The model under review builds one solid part; all positions refer to its coordinate system, in mm. Face numbers are marked on the shaded views. A direction names the side the tool comes from. Give positions to 0.01 mm unless a question says otherwise; leave off trailing zeros. Order: outer loops, then holes, each group sorted by start corner. A loop starts at its lowest first (then second) coordinate and runs counter-clockwise, first axis right, second up. Notation, with made-up numbers: (19.25, 70.5) - (67.25, 70.5) arc R11 cw to (67.25, 84.5) - close; hole circle Ø2 at (-34.75, 47.5). An arc over 180 degrees is marked (long way). Answer as CSV lines item,"result". Start each with the question number.
from build123d import *

# Parameters (mm, degrees)
SKETCH1_W                 = 43
SKETCH1_H                 = 60
BOSS_EXTRUDE1_DEPTH       = 55
SKETCH2_W                 = 41.9
SKETCH2_H                 = 20.5
SKETCH2_H_2               = 20
CUT_EXTRUDE1_DEPTH        = 38
SKETCH3_W                 = 9.05
SKETCH3_H                 = 8.5
CUT_EXTRUDE2_DEPTH        = 38
BOSS_EXTRUDE5_START       = -0.874015748
BOSS_EXTRUDE5_OUTLINE_W   = 2.5
BOSS_EXTRUDE5_OUTLINE_H   = 41.9
BOSS_EXTRUDE5_OUTLINE_W_2 = 5
BOSS_EXTRUDE5_OUTLINE_H_2 = 20
BOSS_EXTRUDE5_DEPTH       = 30
SKETCH18_R                = 2.5
CUT_EXTRUDE9_DEPTH        = 10
SKETCH19_R                = 2.5
CUT_EXTRUDE10_DEPTH       = 10
SKETCH20_W                = 41.9
SKETCH20_H                = 5
CUT_EXTRUDE11_DEPTH       = 25
SKETCH21_W                = 60
SKETCH21_H                = 55
CUT_EXTRUDE12_DEPTH       = 13
SKETCH22_W                = 41.9
SKETCH22_H                = 2
BOSS_EXTRUDE6_DEPTH       = 25
FILLET4_R                 = 1
FILLET5_R                 = 1


# Read off the part's stored shape, not the designer's step: Boss-Extrude5
with BuildPart() as part:
    # Sketch1 → Boss-Extrude1 (new body)
    with BuildSketch(Plane(origin=(0, 0, 0), x_dir=(1, 0, 0), z_dir=(0, 1, 0))):
        with Locations((20.625984252, 7.362204724)):
            Rectangle(SKETCH1_W, SKETCH1_H)
    extrude(amount=BOSS_EXTRUDE1_DEPTH)

    # Sketch2 → Cut-Extrude1 (cut)
    with BuildSketch(Plane(origin=(42.125984252, 0, 0), x_dir=(0, 0, -1), z_dir=(1, 0, 0))):
        with Locations((7.362204724, 40.25)):
            Rectangle(SKETCH2_W, SKETCH2_H)
        with Locations((7.362204724, 14.5)):
            Rectangle(SKETCH2_W, SKETCH2_H_2)
    extrude(amount=-CUT_EXTRUDE1_DEPTH, mode=Mode.SUBTRACT)

    # Sketch3 → Cut-Extrude2 (cut)
    with BuildSketch(Plane(origin=(42.125984252, 0, 0), x_dir=(0, 0, -1), z_dir=(1, 0, 0))):
        with Locations((-18.112795276, 14.75)):
            Rectangle(SKETCH3_W, SKETCH3_H)
        with Locations((32.837204724, 40.25)):
            Rectangle(SKETCH3_W, SKETCH3_H)
    extrude(amount=-CUT_EXTRUDE2_DEPTH, mode=Mode.SUBTRACT)

    # Boss-Extrude5 outline → Boss-Extrude5 (add)
    with BuildSketch(Plane.YZ.offset(BOSS_EXTRUDE5_START)):
        with Locations((5.75, -7.362204724)):
            Rectangle(BOSS_EXTRUDE5_OUTLINE_W, BOSS_EXTRUDE5_OUTLINE_H)
        with Locations((4.5, -47.362204724)):
            Rectangle(BOSS_EXTRUDE5_OUTLINE_W_2, BOSS_EXTRUDE5_OUTLINE_H_2)
        with Locations((4.5, 32.637795276)):
            Rectangle(BOSS_EXTRUDE5_OUTLINE_W_2, BOSS_EXTRUDE5_OUTLINE_H_2)
    extrude(amount=BOSS_EXTRUDE5_DEPTH)

    # Sketch18 → Cut-Extrude9 (cut)
    with BuildSketch(Plane(origin=(29.125984252, 0, 0), x_dir=(0, 0, -1), z_dir=(1, 0, 0))):
        with Locations((-17.437795276, 45.5)):
            Circle(SKETCH18_R)
        with Locations((-17.437795276, 35.5)):
            Circle(SKETCH18_R)
    extrude(amount=-CUT_EXTRUDE9_DEPTH, mode=Mode.SUBTRACT)

    # Sketch19 → Cut-Extrude10 (cut)
    with BuildSketch(Plane(origin=(29.125984252, 0, 0), x_dir=(0, 0, -1), z_dir=(1, 0, 0))):
        with Locations((32.162204724, 19.5)):
            Circle(SKETCH19_R)
        with Locations((32.162204724, 9.5)):
            Circle(SKETCH19_R)
    extrude(amount=-CUT_EXTRUDE10_DEPTH, mode=Mode.SUBTRACT)

    # Sketch20 → Cut-Extrude11 (cut)
    with BuildSketch(Plane(origin=(29.125984252, 0, 0), x_dir=(0, 0, -1), z_dir=(1, 0, 0))):
        with Locations((7.362204724, 4.5)):
            Rectangle(SKETCH20_W, SKETCH20_H)
    extrude(amount=-CUT_EXTRUDE11_DEPTH, mode=Mode.SUBTRACT)

    # Sketch21 → Cut-Extrude12 (cut)
    with BuildSketch(Plane(origin=(42.125984252, 0, 0), x_dir=(0, 0, -1), z_dir=(1, 0, 0))):
        with Locations((7.362204724, 27.5)):
            Rectangle(SKETCH21_W, SKETCH21_H)
    extrude(amount=-CUT_EXTRUDE12_DEPTH, mode=Mode.SUBTRACT)

    # Sketch22 → Boss-Extrude6 (add)
    with BuildSketch(Plane(origin=(4.125984252, 0, 0), x_dir=(0, 0, -1), z_dir=(1, 0, 0))):
        with Locations((7.362204724, 3)):
            Rectangle(SKETCH22_W, SKETCH22_H)
    extrude(amount=BOSS_EXTRUDE6_DEPTH)

    # Fillet4
    fillet4_edges = [part.edges().sort_by_distance(p)[0] for p in [
        (29.125984252, 44.5, -32.837204724),
        (29.125984252, 36, -32.837204724),
        (16.625984252, 36, -28.312204724),
        (16.625984252, 44.5, -28.312204724),
        (16.625984252, 44.5, -37.362204724),
        (16.625984252, 36, -37.362204724),
    ]]
    fillet(fillet4_edges, radius=FILLET4_R)

    # Fillet5
    fillet5_edges = [part.edges().sort_by_distance(p)[0] for p in [
        (29.125984252, 10.5, 18.112795276),
        (16.625984252, 10.5, 22.637795276),
        (16.625984252, 10.5, 13.587795276),
    ]]
    fillet(fillet5_edges, radius=FILLET5_R)


solid = part.part
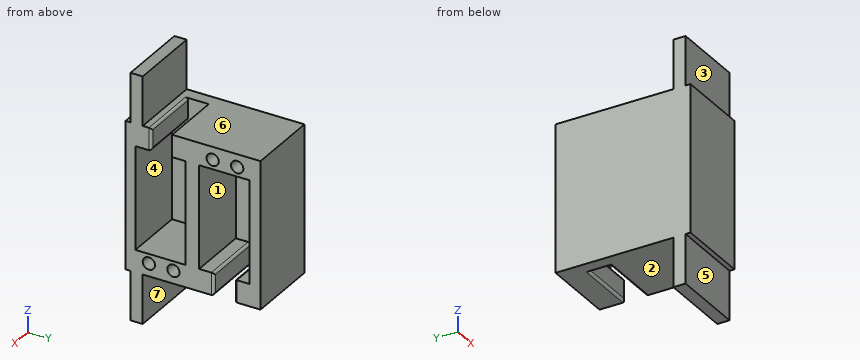
Item 1: Take a section at A-A on y = 5. Write out the cut boundary in (x, z).
Item 2: For line 1 along Y through (x, z) = (12, -20); line 2 along Z through (x, y) = (13, 21.5); line 3 along Z through (x, y) = (25, 9), list the stretches that pass through material, from the lowest coordinate up.
Item 3: Mouldability with a two-part tool opening along Y and no side actions: class the marked faces 1, 2 and 3 as released by +Y, released by -Y, zero draft, split by the parting line, or undercut.
Item 4: Clearance check with flat-ended pins moving along their axes: pin 1 (5 mm diameter, centred on x = 9.5, z = 2.5, fed in from -Y); pin 2 (6 mm diameter, centred on y = 7.5, z = 5.5, fed in from +X); pin 3 (10 mm diameter, centred on x = 10.5, y = 38.5, fed in from -Z); pin 4 (6 mm diameter, centred on x = 13, z = 35.5, fed in from +Y). State where each tip first meets the part, or that it passes through.
Item 5: Take a section at D-D on x = 27. Count the separate pieces of the cut face and the enclosed holes in it, and give its area (3 significant figures).
Item 6: Machinability: for the marked faces 4, 5, 6 and 7, which of the approach directions +Z, -Z, +X, -X, +Y, -Y give a long, thin tool a straight path to every point of the face, cutting with its end or side? Answer none if there is none.
Item 7: Take a section at B-B on z = -1.5. Write out the cut boundary in (x, y).
Data:
1,outline,"(-0.87, -57.36) - (29.13, -57.36) - (29.13, -28.31) - (4.13, -28.31) - (4.13, 13.59) - (29.13, 13.59) - (29.13, 42.64) - (-0.87, 42.64) - close"
2,line 1,"y = 0 to 4, 24.5 to 30, 50.5 to 55"
2,line 2,"z = -37.36 to -28.31, 13.59 to 22.64"
2,line 3,"z = -37.36 to -34.61, -29.71 to -28.31, 13.59 to 22.64"
3,face 1,"undercut"
3,face 2,"zero draft"
3,face 3,"released by -Y"
4,pin 1,"stops at y = 0"
4,pin 2,"stops at x = 4.13"
4,pin 3,"stops at z = -37.36"
4,pin 4,"stops at y = 7"
5,separate pieces,"1"
5,enclosed holes,"4"
5,area,"1,550 mm^2"
6,face 4,"+X"
6,face 5,"-Z, +X, -X, -Y"
6,face 6,"+Z, +X, -X, +Y"
6,face 7,"-Z, +X, -X, +Y"
7,outline,"(-0.87, 0) - (29.13, 0) - (29.13, 4) - (4.13, 4) - (4.13, 24.5) - (29.13, 24.5) - (29.13, 30) - (4.13, 30) - (4.13, 50.5) - (29.13, 50.5) - (29.13, 55) - (-0.87, 55) - close"
